from build123d import *

# Parameters (mm, degrees)
F0_W     = 120
F0_H     = 80
F1_DEPTH = 5
F3_D     = 11
F4_D     = 20
F5_SIZE  = 10


with BuildPart() as f1:
    # F0 (on Top) → F1 (new body, symmetric)
    with BuildSketch(Plane.XY):
        Rectangle(F0_W, F0_H)
    extrude(amount=F1_DEPTH, both=True)

    # F3 (through all)
    with Locations(Plane.XY.offset(5)):
        with Locations((-45, 25), (45, 25), (45, -25), (-45, -25)):
            Hole(F3_D / 2)

    # F4 (through all)
    with Locations(Plane.XY.offset(5)):
        with Locations((0, 0)):
            Hole(F4_D / 2)

    # F5
    f5_edges = [f1.edges().sort_by_distance(p)[0] for p in [
        (-60, -40, 0),
        (-60, 40, 0),
        (60, -40, 0),
        (60, 40, 0),
    ]]
    chamfer(f5_edges, length=F5_SIZE)


solid = f1.part
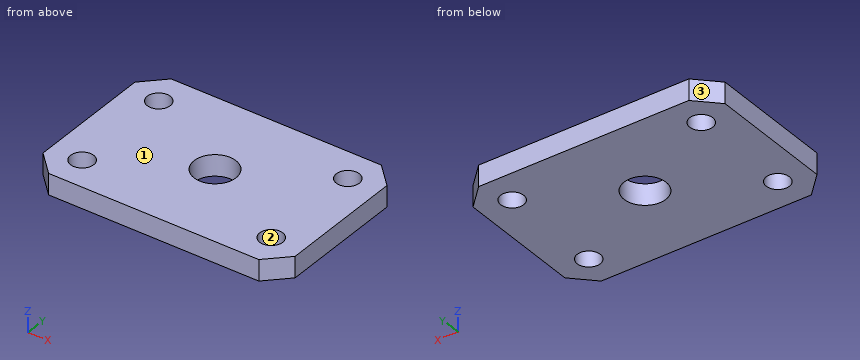
The listing builds one solid part. Answer for the finished solid, in the listing's coordinates (mm). Face numbers are marked on the shaded views. Give positions to 0.01 mm unless a question says otherwise; leave off trailing zeros. Order: outer loops, then holes, each group sorted by start corner. A loop starts at its lowest first (then second) coordinate and runs counter-clockwise, first axis right, second up. Notation, with made-up numbers: (-28.5, -19.5) - (-22.5, -19.5) arc R21 cw to (-22.5, -14.5) - close; hole circle Ø11 at (0.25, -1). An arc over 180 degrees is marked (long way). One line per item, written item: value. Start each with the question number.
1) A cutting plane is placed at A-A on x = -45. Give the vertices of the cut face in (y, z), then the cut area to 3 significant figures.
2) Find the intervals of material crossed by L1, parallel to Y at x = 45, z = 0.5; L2, parallel to X at y = 25.5, z = -3.5; L3, parallel to Y at x = 0, z = 1.5, in increasing order.
3) A cutting plane is placed at D-D on y = 0. Give the vertices of the cut face in (x, z), then the cut area to 3 significant figures.
4) A cutting plane is placed at C-C on z = -3. Give the vertices of the cut face in (x, y), then the cut area to 3 significant figures.
5) A cutting plane is placed at B-B on y = -25. Give the vertices of the cut face in (x, z).
6) The mould has two halves that part along X. Classify the marked faces 1, 2 and 3: released by +X, released by -X, zero draft, split by the parting line, or undercut.
Answer sheet:
1. outline: (-40, -5) - (-30.5, -5) - (-30.5, 5) - (-40, 5) - close; (-19.5, -5) - (19.5, -5) - (19.5, 5) - (-19.5, 5) - close; (30.5, -5) - (40, -5) - (40, 5) - (30.5, 5) - close
1. area: 580 mm2
2. L1: y = -40 to -30.5, -19.5 to 19.5, 30.5 to 40
2. L2: x = -60 to -50.48, -39.52 to 39.52, 50.48 to 60
2. L3: y = -40 to -10, 10 to 40
3. outline: (-60, -5) - (-10, -5) - (-10, 5) - (-60, 5) - close; (10, -5) - (60, -5) - (60, 5) - (10, 5) - close
3. area: 1,000 mm2
4. outline: (-60, -30) - (-50, -40) - (50, -40) - (60, -30) - (60, 30) - (50, 40) - (-50, 40) - (-60, 30) - close; hole circle Ø11 at (-45, -25); hole circle Ø11 at (-45, 25); hole circle Ø20 at (0, 0); hole circle Ø11 at (45, -25); hole circle Ø11 at (45, 25)
4. area: 8,710 mm2
5. outline: (-60, -5) - (-50.5, -5) - (-50.5, 5) - (-60, 5) - close; (-39.5, -5) - (39.5, -5) - (39.5, 5) - (-39.5, 5) - close; (50.5, -5) - (60, -5) - (60, 5) - (50.5, 5) - close
6. face 1: zero draft
6. face 2: undercut
6. face 3: released by -X
